Job drawing, mm, ordinate dimensions from the low corner. One solid piece. Give positions to 0.01 mm unless a question says otherwise; leave off trailing zeros. Write each loop counter-clockwise with the first axis right and the second up, starting at its lowest first coordinate (ties: lowest second). Pieces come first, ordered by that corner, then holes. Notation, with made-up numbers: (89, 69) - (129, 69) arc R15 cw to (129, 80) - close; hole circle Ø11 at (47, 8). An arc over 180 degrees is marked (long way). Use a Markdown table: item, result. Add a question column.
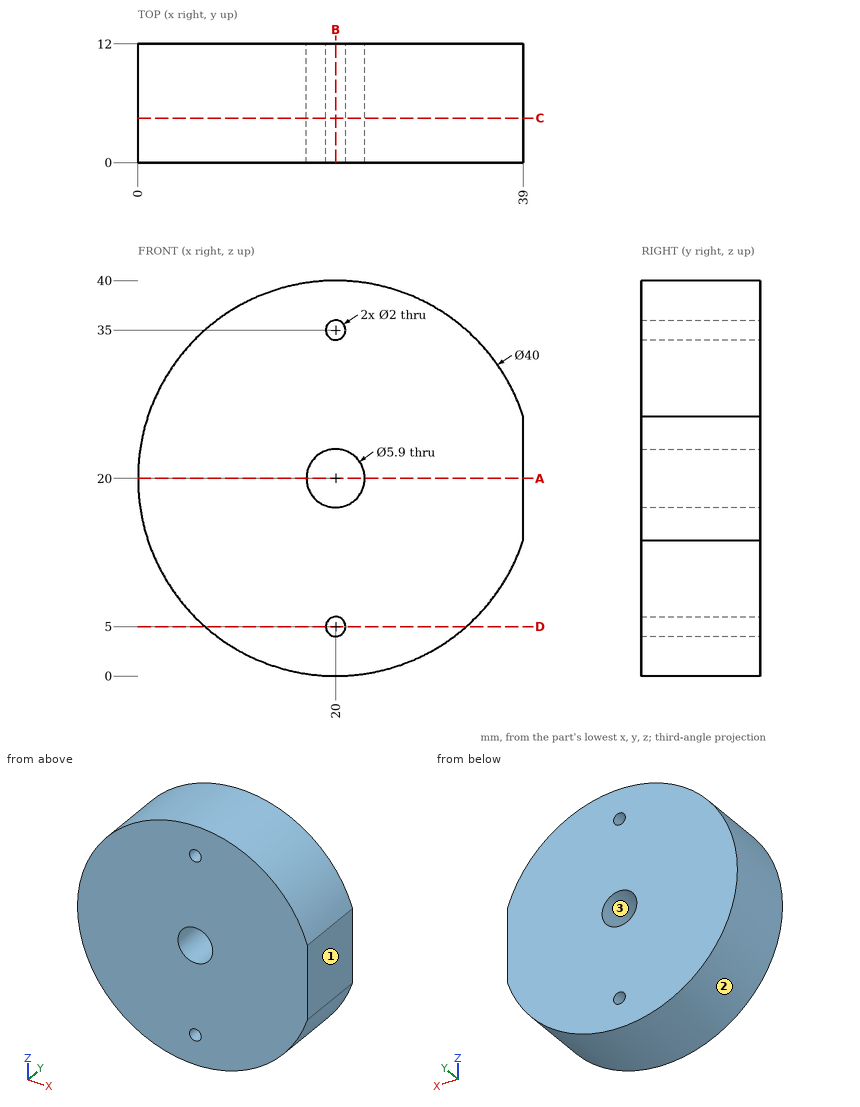
(1) Band-saw the part on C-C (y = 4.5). Write the cut outline in (x, z) (3 decimals).
(2) Two-plate mould, pull along X, no slides. Class the marked faces 1, 2 and 3: +X half, -X half, draft (parallel to the pull), parting line (faces both ways), or undercut.
(3) Band-saw the part on A-A (z = 20). Write the cut outline in (x, y).
(4) Band-saw the part on B-B (x = 20). Write the cut outline in (y, z).
(5) Band-saw the part on D-D (z = 5). Write the cut outline in (x, y), then the cut area to 3 significant figures.
(6) Flat gauge pins, fed straight in: pin 1 (6 mm diameter, centred on y = 6.5, z = 33, fed in from -X); pin 2 (6 mm diameter, centred on y = 3.5, z = 32.5, fed in from +X); pin 3 (6 mm diameter, centred on y = 3.5, z = 21.5, fed in from -X). Where does each tip first touch, or does it go through?
(7) Probe probe 1 along Z at (x, y) = (20, 5.25); probe 2 along Z at (x, y) = (22.5, 6.5); probe 3 along Z at (x, y) = (32, 4.5). List the from-to ranges inside material, lowest first. Write a range as [from, to].
Model answer:
| question | item | result |
|---|---|---|
| 1 | outline | (39, 13.755) - (39, 26.245) arc R20 ccw (long way) to start; hole circle Ø5.9 at (20, 20); hole circle Ø2 at (20, 5); hole circle Ø2 at (20, 35) |
| 2 | face 1 | +X half |
| 2 | face 2 | parting line |
| 2 | face 3 | undercut |
| 3 | outline | (0, 0) - (17.05, 0) - (17.05, 12) - (0, 12) - close; (22.95, 0) - (39, 0) - (39, 12) - (22.95, 12) - close |
| 4 | outline | (0, 0) - (12, 0) - (12, 4) - (0, 4) - close; (0, 6) - (12, 6) - (12, 17.05) - (0, 17.05) - close; (0, 22.95) - (12, 22.95) - (12, 34) - (0, 34) - close; (0, 36) - (12, 36) - (12, 40) - (0, 40) - close |
| 5 | outline | (6.77, 0) - (19, 0) - (19, 12) - (6.77, 12) - close; (21, 0) - (33.23, 0) - (33.23, 12) - (21, 12) - close |
| 5 | area | 293 mm^2 |
| 6 | pin 1 | stops at x = 2.68 |
| 6 | pin 2 | stops at x = 37.6 |
| 6 | pin 3 | stops at x = 0 |
| 7 | probe 1 | z = [0, 4], [6, 17.05], [22.95, 34], [36, 40] |
| 7 | probe 2 | z = [0.16, 18.43], [21.57, 39.84] |
| 7 | probe 3 | z = [4, 36] |
